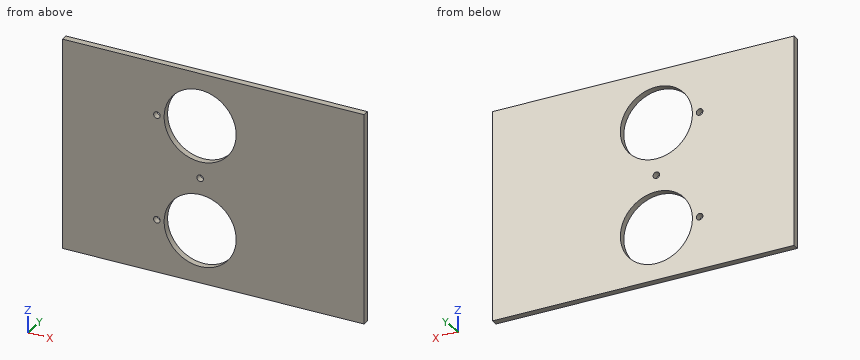
```python
from build123d import *

# Parameters (mm, degrees)
SKETCH_1_W          = 250
SKETCH_1_H          = 160
EXTRUDE_1_DEPTH     = 5
CUT_EXTRUDE_1_REACH = 150.492
SKETCH_2_R          = 27.5
SKETCH_2_R_2        = 2.5
SKETCH_2_W          = 40
SKETCH_2_H          = 160


with BuildPart() as part:
    # 草图1 → 凸台-拉伸1 (new body)
    with BuildSketch(Plane(origin=(0, 0, 0), x_dir=(1, 0, 0), z_dir=(0, 1, 0))):
        Rectangle(SKETCH_1_W, SKETCH_1_H)
    extrude(amount=EXTRUDE_1_DEPTH)

    # 草图2 → 切除-拉伸1 (cut, up to next)
    with BuildSketch(Plane.XZ, mode=Mode.PRIVATE) as cut_extrude_1_sk1:
        with Locations(Location((0, -40, 0), (0, 0, 270))):
            Circle(SKETCH_2_R)
    cut_extrude_1_tool1 = extrude(cut_extrude_1_sk1.sketch, amount=-CUT_EXTRUDE_1_REACH, mode=Mode.PRIVATE) & part.part
    # 草图2 → 切除-拉伸1 (cut, up to next)
    with BuildSketch(Plane.XZ, mode=Mode.PRIVATE) as cut_extrude_1_sk2:
        with Locations(Location((-33, -40, 0), (0, 0, 270))):
            Circle(SKETCH_2_R_2)
    cut_extrude_1_tool2 = extrude(cut_extrude_1_sk2.sketch, amount=-CUT_EXTRUDE_1_REACH, mode=Mode.PRIVATE) & part.part
    # 草图2 → 切除-拉伸1 (cut, up to next)
    with BuildSketch(Plane.XZ, mode=Mode.PRIVATE) as cut_extrude_1_sk3:
        with Locations(Location((-33, 40, 0), (0, 0, 270))):
            Circle(SKETCH_2_R_2)
    cut_extrude_1_tool3 = extrude(cut_extrude_1_sk3.sketch, amount=-CUT_EXTRUDE_1_REACH, mode=Mode.PRIVATE) & part.part
    # 草图2 → 切除-拉伸1 (cut, up to next)
    with BuildSketch(Plane.XZ, mode=Mode.PRIVATE) as cut_extrude_1_sk4:
        with Locations(Location((0, 40, 0), (0, 0, 270))):
            Circle(SKETCH_2_R)
    cut_extrude_1_tool4 = extrude(cut_extrude_1_sk4.sketch, amount=-CUT_EXTRUDE_1_REACH, mode=Mode.PRIVATE) & part.part
    # 草图2 → 切除-拉伸1 (cut, up to next)
    with BuildSketch(Plane.XZ, mode=Mode.PRIVATE) as cut_extrude_1_sk5:
        with Locations(Location((0, 0, 0), (0, 0, 270))):
            Circle(SKETCH_2_R_2)
    cut_extrude_1_tool5 = extrude(cut_extrude_1_sk5.sketch, amount=-CUT_EXTRUDE_1_REACH, mode=Mode.PRIVATE) & part.part
    # 草图2 → 切除-拉伸1 (cut, up to next)
    with BuildSketch(Plane.XZ, mode=Mode.PRIVATE) as cut_extrude_1_sk6:
        with Locations((-125, 0)):
            Rectangle(SKETCH_2_W, SKETCH_2_H)
    cut_extrude_1_tool6 = extrude(cut_extrude_1_sk6.sketch, amount=-CUT_EXTRUDE_1_REACH, mode=Mode.PRIVATE) & part.part
    add(cut_extrude_1_tool1.solids().sort_by_distance((0, 0, -40))[0], mode=Mode.SUBTRACT)
    add(cut_extrude_1_tool2.solids().sort_by_distance((-33, 0, -40))[0], mode=Mode.SUBTRACT)
    add(cut_extrude_1_tool3.solids().sort_by_distance((-33, 0, 40))[0], mode=Mode.SUBTRACT)
    add(cut_extrude_1_tool4.solids().sort_by_distance((0, 0, 40))[0], mode=Mode.SUBTRACT)
    add(cut_extrude_1_tool5.solids().sort_by_distance((0, 0, 0))[0], mode=Mode.SUBTRACT)
    add(cut_extrude_1_tool6.solids().sort_by_distance((-125, 0, 0))[0], mode=Mode.SUBTRACT)


solid = part.part
```
The model under review builds one solid part; all positions refer to its coordinate system, in mm. Round coordinates to 2 decimals unless told otherwise and drop trailing zeros. Order: outer loops, then holes, each group sorted by start corner. A loop starts at its lowest first (then second) coordinate and runs counter-clockwise, first axis right, second up.
(1) Take a section at C-C, the plane x = -24.5. State the section outline as (y, z) points.
Working result:
outline: (0, -80) - (5, -80) - (5, -52.49) - (0, -52.49) - close; (0, -27.51) - (5, -27.51) - (5, 27.51) - (0, 27.51) - close; (0, 52.49) - (5, 52.49) - (5, 80) - (0, 80) - close
(2) Take a section at B-B, the plane z = -40. State the section outline as (x, y) points, plus the area to 3 significant figures.
Working result:
outline: (-105, 0) - (-35.5, 0) - (-35.5, 5) - (-105, 5) - close; (-30.5, 0) - (-27.5, 0) - (-27.5, 5) - (-30.5, 5) - close; (27.5, 0) - (125, 0) - (125, 5) - (27.5, 5) - close
area: 850 mm2
(3) Wall thickness on L1, parallel to X at y = 3.8, z = 40; L2, parallel to Z at x = 12.5, y = 3.8; L3, parallel to X at y = 3.85, z = 0: over which ranges is each line inside the solid? List them lowest first.
Working result:
L1: x = -105 to -35.5, -30.5 to -27.5, 27.5 to 125
L2: z = -80 to -64.49, -15.51 to 15.51, 64.49 to 80
L3: x = -105 to -2.5, 2.5 to 125
(4) Take a section at D-D, the plane z = 0. State the section outline as (x, y) points, plus the area to 4 significant figures.
Working result:
outline: (-105, 0) - (-2.5, 0) - (-2.5, 5) - (-105, 5) - close; (2.5, 0) - (125, 0) - (125, 5) - (2.5, 5) - close
area: 1,125 mm2
(5) Take a section at A-A, the plane x = 0. State the section outline as (y, z) points.
Working result:
outline: (0, -80) - (5, -80) - (5, -67.5) - (0, -67.5) - close; (0, -12.5) - (5, -12.5) - (5, -2.5) - (0, -2.5) - close; (0, 2.5) - (5, 2.5) - (5, 12.5) - (0, 12.5) - close; (0, 67.5) - (5, 67.5) - (5, 80) - (0, 80) - close
